Input: part model. Units: mm. Frame: model coordinates. A direction names the side the tool comes from. Give positions to 0.01 mm unless a question says otherwise; leave off trailing zeros. One line per item, written item: value.
from build123d import *

# Parameters (mm, degrees)
SKETCH1_W           = 2108.2
SKETCH1_H           = 184.15
BOSS_EXTRUDE1_DEPTH = 22.225
CUT_EXTRUDE2_START  = -22.225
SKETCH2_R           = 13.4874
CUT_EXTRUDE2_DEPTH  = 88.9
CUT_EXTRUDE4_START  = -22.225
SKETCH3_R           = 19.8374
CUT_EXTRUDE4_DEPTH  = 25.4
CUT_EXTRUDE6_START  = -22.225
SKETCH4_R           = 13.4874
CUT_EXTRUDE6_DEPTH  = 88.9
CUT_EXTRUDE8_START  = -22.225
SKETCH5_R           = 19.8374
CUT_EXTRUDE8_DEPTH  = 25.4
CHAMFER1_SIZE       = 1.524


with BuildPart() as part:
    # Sketch1 → Boss-Extrude1 (new, symmetric)
    with BuildSketch(Plane(origin=(0, 0, 0), x_dir=(1, 0, 0), z_dir=(0, 1, 0))):
        Rectangle(SKETCH1_W, SKETCH1_H)
    extrude(amount=BOSS_EXTRUDE1_DEPTH, both=True)

    # Sketch2 → Cut-Extrude2 (cut)
    with BuildSketch(Plane(origin=(0, 0, 0), x_dir=(1, 0, 0), z_dir=(0, 1, 0)).offset(CUT_EXTRUDE2_START)):
        with Locations(Location((-1016, -60.325, 0), (0, 0, 90))):
            Circle(SKETCH2_R)
        with Locations(Location((-508, -60.325, 0), (0, 0, 90))):
            Circle(SKETCH2_R)
        with Locations(Location((0, -60.325, 0), (0, 0, 90))):
            Circle(SKETCH2_R)
        with Locations(Location((508, -60.325, 0), (0, 0, 90))):
            Circle(SKETCH2_R)
        with Locations(Location((1016, -60.325, 0), (0, 0, 90))):
            Circle(SKETCH2_R)
    extrude(amount=CUT_EXTRUDE2_DEPTH, mode=Mode.SUBTRACT)

    # Sketch3 → Cut-Extrude4 (cut)
    with BuildSketch(Plane(origin=(0, 0, 0), x_dir=(1, 0, 0), z_dir=(0, 1, 0)).offset(CUT_EXTRUDE4_START)):
        with Locations(Location((-1016, -60.325, 0), (0, 0, 270))):
            Circle(SKETCH3_R)
        with Locations(Location((-508, -60.325, 0), (0, 0, 270))):
            Circle(SKETCH3_R)
        with Locations(Location((0, -60.325, 0), (0, 0, 270))):
            Circle(SKETCH3_R)
        with Locations(Location((508, -60.325, 0), (0, 0, 270))):
            Circle(SKETCH3_R)
        with Locations(Location((1016, -60.325, 0), (0, 0, 270))):
            Circle(SKETCH3_R)
    extrude(amount=CUT_EXTRUDE4_DEPTH, mode=Mode.SUBTRACT)

    # Sketch4 → Cut-Extrude6 (cut)
    with BuildSketch(Plane(origin=(0, 0, 0), x_dir=(1, 0, 0), z_dir=(0, 1, 0)).offset(CUT_EXTRUDE6_START)):
        with Locations(Location((-762, -15.875, 0), (0, 0, 90))):
            Circle(SKETCH4_R)
        with Locations(Location((-254, -15.875, 0), (0, 0, 90))):
            Circle(SKETCH4_R)
        with Locations(Location((254, -15.875, 0), (0, 0, 90))):
            Circle(SKETCH4_R)
        with Locations(Location((762, -15.875, 0), (0, 0, 90))):
            Circle(SKETCH4_R)
    extrude(amount=CUT_EXTRUDE6_DEPTH, mode=Mode.SUBTRACT)

    # Sketch5 → Cut-Extrude8 (cut)
    with BuildSketch(Plane(origin=(0, 0, 0), x_dir=(1, 0, 0), z_dir=(0, 1, 0)).offset(CUT_EXTRUDE8_START)):
        with Locations(Location((-762, -15.875, 0), (0, 0, 270))):
            Circle(SKETCH5_R)
        with Locations(Location((-254, -15.875, 0), (0, 0, 270))):
            Circle(SKETCH5_R)
        with Locations(Location((254, -15.875, 0), (0, 0, 270))):
            Circle(SKETCH5_R)
        with Locations(Location((762, -15.875, 0), (0, 0, 270))):
            Circle(SKETCH5_R)
    extrude(amount=CUT_EXTRUDE8_DEPTH, mode=Mode.SUBTRACT)

    # Chamfer1
    chamfer1_edges = [part.edges().sort_by_distance(p)[0] for p in [
        (0, -22.225, -92.075),
        (0, 22.225, -92.075),
    ]]
    chamfer(chamfer1_edges, length=CHAMFER1_SIZE)


solid = part.part
Item 1: Access query for faces 3 (the face through (-15, 22.225, -1)), 4 (the face through (775.407, -9.703, 1.254)). Directions: +Z, -Z, +X, -X, +Y, -Y. A direction counts if a zero-diameter tool reaches every point of the face in a straight line with its end or side. Return the directions, or none.
Verdict:
face 3: +Z, -Z, +X, -X, +Y
face 4: -Y
Item 2: Material intervals for L1, parallel to X at y = 10, z = 25; L2, parallel to X at y = -10, z = 4; L3, parallel to Z at x = 501, y = 16 (3 decimals), sorted ascending.
Verdict:
L1: x = -1054.1 to -771.93, -752.07 to -263.93, -244.07 to 244.07, 263.93 to 752.07, 771.93 to 1054.1
L2: x = -1054.1 to -777.89, -746.11 to -269.89, -238.11 to 238.11, 269.89 to 746.11, 777.89 to 1054.1
L3: z = -92.075 to 48.796, 71.854 to 92.075
Item 3: Draft query along X for faces 1 (the face through (-15, 0, 92.075)), 2 (the face through (-234.33, -9.7, 13.29)). Return one class per face: pulls with the +X half, pulls with the -X half, needs draft (parallel to the pull), parting line crosses it, or undercut.
Verdict:
face 1: needs draft
face 2: undercut
